Verification items for the finished model (mm, model axes). Face numbers are marked on the shaded views. A direction names the side the tool comes from. Coordinates: 2 decimals unless noted, no trailing zeros. Loops run counter-clockwise (first coordinate to the right, second up) from the corner with the lowest first, then second, coordinate; pieces in that order, holes last.
Q1. Mould release check, pull along Y, two halves, no side actions. Record for the marked faces 5, 6 and 7: +Y half, -Y half, draft (parallel to the pull), parting line (faces both ways), or undercut.
Q2. Access from +Z, -Z, +X, -X, +Y, -Y to the whole of each face (thin tool, end or side, straight path). Record for the marked faces 1, 2, 3 and 4.
Q3. Sectioned sample at C-C (y = 237.5). Enter the section's corners in (x, z), then the cut area to 3 significant figures.
Q4. Go/stop test with flat-tipped pins: P1, Ø0.9, axis at y = 267, z = 1.5, coming from the +X side; P2, Ø0.5, axis at y = 221.5, z = 2, coming from the -X side; P3, Ø0.9, axis at x = 132.45, y = 223.12, coming from the -Z side; P4, Ø1.5, axis at x = 138, z = 2, coming from the +Y side. Record where each tip stops, or that it passes through.
Q5. Material ranges on probe 1 along Y at (x, z) = (165, 0.9); probe 2 along X at (y, z) = (257, 0.8); probe 3 along Y at (x, z) = (126.5, 2.25), recorded low to high.
Q6. Sectioned sample at D-D (x = 140.5). Enter the section's corners in (y, z).
Q7. Sectioned sample at B-B (y = 227). Enter the section's corners in (x, z), then the cut area to 3 significant figures.
Q8. Sectioned sample at A-A (x = 166). Enter the section's corners in (y, z), then the cut area to 3 significant figures.
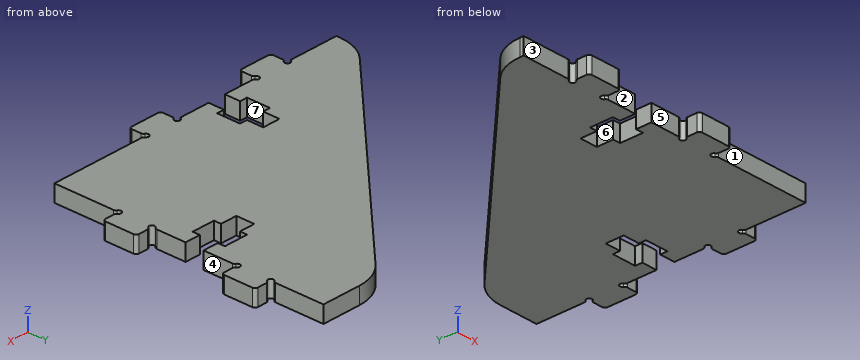
```python
from build123d import *

# Parameters (mm, degrees)
BOSS_EXTRUDE1_DEPTH = 3


with BuildPart() as part:
    # Sketch1 → Boss-Extrude1 (new body)
    with BuildSketch(Plane.XY):
        with BuildLine():
            Line((154.202092406, 220.554881742), (154.202092406, 222.231534508))
            ThreePointArc((154.202092406, 222.231534508), (154.133358076, 222.488056371), (153.945571469, 222.675843656))
            ThreePointArc((153.945571469, 222.675843656), (153.839317887, 223.482927965), (154.646402272, 223.376674963))
            ThreePointArc((154.646402272, 223.376674963), (154.834188461, 223.188888947), (155.090708914, 223.120153964))
            Line((155.090708914, 223.120153964), (172.247320861, 223.120153964))
            Line((172.247320861, 223.120153964), (172.247320861, 233.928920262))
            ThreePointArc((172.247320861, 233.928920262), (172.178586068, 234.185442001), (171.990799121, 234.373228947))
            ThreePointArc((171.990799121, 234.373228947), (171.884544083, 235.180313064), (172.69162866, 235.074061519))
            ThreePointArc((172.69162866, 235.074061519), (172.879415632, 234.886275586), (173.135936791, 234.817541323))
            Line((173.135936791, 234.817541323), (174.812591608, 234.817541323))
            ThreePointArc((174.812591608, 234.817541323), (175.175368126, 234.96780829), (175.325635071, 235.330584817))
            Line((175.325635071, 235.330584817), (175.325635071, 240.461016521))
            ThreePointArc((175.325635071, 240.461016521), (175.175368781, 240.82379332), (174.812592535, 240.974060941))
            Line((174.812592535, 240.974060941), (173.135939769, 240.974060941))
            ThreePointArc((173.135939769, 240.974060941), (172.879418072, 240.905325991), (172.691631242, 240.717538929))
            ThreePointArc((172.691631242, 240.717538929), (171.88454719, 240.611283394), (171.990798239, 241.418368036))
            ThreePointArc((171.990798239, 241.418368036), (172.178584056, 241.606155124), (172.247318162, 241.862676325))
            Line((172.247318162, 241.862676325), (172.247318162, 247.130575977))
            Line((172.247318162, 247.130575977), (169.447318162, 247.130575977))
            Line((169.447318162, 247.130575977), (169.447318162, 245.822321264))
            Line((169.447318162, 245.822321264), (165.247318162, 245.822321264))
            Line((165.247318162, 245.822321264), (165.247318162, 247.130575977))
            Line((165.247318162, 247.130575977), (162.247318162, 247.130575977))
            Line((162.247318162, 247.130575977), (162.247318162, 250.414066551))
            Line((162.247318162, 250.414066551), (165.064709466, 250.414066551))
            Line((165.064709466, 250.414066551), (165.064709466, 251.722321264))
            Line((165.064709466, 251.722321264), (169.447318162, 251.722321264))
            Line((169.447318162, 251.722321264), (169.447318162, 250.414066551))
            Line((169.447318162, 250.414066551), (172.247318162, 250.414066551))
            Line((172.247318162, 250.414066551), (172.247318162, 255.681968256))
            ThreePointArc((172.247318162, 255.681968256), (172.178583369, 255.938489995), (171.990796423, 256.126276941))
            ThreePointArc((171.990796423, 256.126276941), (171.884540761, 256.933361837), (172.691625961, 256.827108487))
            ThreePointArc((172.691625961, 256.827108487), (172.879412934, 256.639322554), (173.135934092, 256.57058829))
            Line((173.135934092, 256.57058829), (174.81258891, 256.57058829))
            ThreePointArc((174.81258891, 256.57058829), (175.175365428, 256.720855257), (175.325632372, 257.083631785))
            Line((175.325632372, 257.083631785), (175.325632372, 262.214063489))
            ThreePointArc((175.325632372, 262.214063489), (175.175366082, 262.576840287), (174.812589836, 262.727107909))
            Line((174.812589836, 262.727107909), (173.135937071, 262.727107909))
            ThreePointArc((173.135937071, 262.727107909), (172.879415358, 262.658373018), (172.691628483, 262.470586))
            ThreePointArc((172.691628483, 262.470586), (171.884544407, 262.364330653), (171.990795644, 263.17141527))
            ThreePointArc((171.990795644, 263.17141527), (172.178581505, 263.359202315), (172.24731567, 263.6157235))
            Line((172.24731567, 263.6157235), (172.24731567, 272.372324682))
            Line((172.24731567, 272.372324682), (165.195283942, 272.372324682))
            ThreePointArc((165.195283942, 272.372324682), (162.053952222, 271.747474765), (159.390859837, 269.968053135))
            Line((159.390859837, 269.968053135), (119.051573553, 229.628769332))
            ThreePointArc((119.051573553, 229.628769332), (117.272153027, 226.965676711), (116.647304057, 223.824345228))
            Line((116.647304057, 223.824345228), (116.647304057, 223.120152431))
            Line((116.647304057, 223.120152431), (125.403905518, 223.120152431))
            ThreePointArc((125.403905518, 223.120152431), (125.660427257, 223.188887224), (125.848214203, 223.37667417))
            ThreePointArc((125.848214203, 223.37667417), (126.655299099, 223.482929832), (126.549045749, 222.675844632))
            ThreePointArc((126.549045749, 222.675844632), (126.361259816, 222.488057659), (126.292525553, 222.231536501))
            Line((126.292525553, 222.231536501), (126.292525553, 220.554881683))
            ThreePointArc((126.292525553, 220.554881683), (126.442792519, 220.192105166), (126.805569047, 220.041838221))
            Line((126.805569047, 220.041838221), (131.936000751, 220.041838221))
            ThreePointArc((131.936000751, 220.041838221), (132.298776762, 220.192104665), (132.449044229, 220.554880252))
            Line((132.449044229, 220.554880252), (132.449044229, 222.231533018))
            ThreePointArc((132.449044229, 222.231533018), (132.380309899, 222.488054881), (132.192523292, 222.675842166))
            ThreePointArc((132.192523292, 222.675842166), (132.08626971, 223.482926475), (132.893354095, 223.376673473))
            ThreePointArc((132.893354095, 223.376673473), (133.081140729, 223.188887201), (133.337661764, 223.120152474))
            Line((133.337661764, 223.120152474), (138.647308242, 223.120152474))
            Line((138.647308242, 223.120152474), (138.647308242, 225.920152474))
            Line((138.647308242, 225.920152474), (137.297308242, 225.920152474))
            Line((137.297308242, 225.920152474), (137.297308242, 230.120152474))
            Line((137.297308242, 230.120152474), (138.647308242, 230.120152474))
            Line((138.647308242, 230.120152474), (138.647308242, 233.120152474))
            Line((138.647308242, 233.120152474), (141.847308242, 233.120152474))
            Line((141.847308242, 233.120152474), (141.847308242, 230.120152474))
            Line((141.847308242, 230.120152474), (143.197308242, 230.120152474))
            Line((143.197308242, 230.120152474), (143.197308242, 225.920152474))
            Line((143.197308242, 225.920152474), (141.847308242, 225.920152474))
            Line((141.847308242, 225.920152474), (141.847308242, 223.120152474))
            Line((141.847308242, 223.120152474), (147.156952668, 223.120152474))
            ThreePointArc((147.156952668, 223.120152474), (147.413474407, 223.188887267), (147.601261354, 223.376674213))
            ThreePointArc((147.601261354, 223.376674213), (148.408346249, 223.482929875), (148.302092899, 222.675844675))
            ThreePointArc((148.302092899, 222.675844675), (148.114306966, 222.488057703), (148.045572703, 222.231536544))
            Line((148.045572703, 222.231536544), (148.045572703, 220.554881727))
            ThreePointArc((148.045572703, 220.554881727), (148.19583967, 220.192105209), (148.558616197, 220.041838264))
            Line((148.558616197, 220.041838264), (153.689048927, 220.041838264))
            ThreePointArc((153.689048927, 220.041838264), (154.05182545, 220.19210522), (154.202092406, 220.554881742))
        make_face()
    extrude(amount=BOSS_EXTRUDE1_DEPTH)


solid = part.part
```
Geometry check:
1. face 5: -Y half
1. face 6: draft
1. face 7: undercut
2. face 1: +Z, -Z, +X, -Y
2. face 2: +Z, -Z, -Y
2. face 3: +Z, -Z, -X, -Y
2. face 4: +Z, -Z, +X
3. outline: (126.92, 0) - (175.33, 0) - (175.33, 3) - (126.92, 3) - close
3. area: 145 mm2
4. P1: stops at x = 172.25
4. P2: stops at x = 126.29
4. P3: passes through
4. P4: stops at y = 249.33
5. probe 1: y = 223.12 to 247.13, 250.41 to 272.37
5. probe 2: x = 146.42 to 171.97, 172.53 to 175.32
5. probe 3: y = 220.14 to 222.64, 223.59 to 237.08
6. outline: (233.12, 0) - (251.08, 0) - (251.08, 3) - (233.12, 3) - close
7. outline: (117.29, 0) - (137.3, 0) - (137.3, 3) - (117.29, 3) - close; (143.2, 0) - (172.25, 0) - (172.25, 3) - (143.2, 3) - close
7. area: 147 mm2
8. outline: (223.12, 0) - (245.82, 0) - (245.82, 3) - (223.12, 3) - close; (251.72, 0) - (272.37, 0) - (272.37, 3) - (251.72, 3) - close
8. area: 130 mm2
